Autodesk Inventor part; units mm, degrees
ref_plane "Arbeitsebene1" through (0, 0, 0) normal (0, 1, 0) x (-1, 0, 0)
ref_plane "YZ Plane" through (0, 0, 0) normal (1, 0, 0) x (0, 1, 0)
ref_plane "XY Plane" through (0, 0, 0) normal (0, 0, 1) x (1, 0, 0)
sketch "Skizze1" plane through (0, 0, 0) normal (0, 0, 1) x (1, 0, 0)
  line L0 (-2.6307, 4) -> (27.3693, 4) construction
  arc A0 (0, 0) -> (24.7386, 0) centre (12.3693, 4) ccw
  circle A1 centre (12.3693, 4) radius 5.5
  line L1 (17.8693, 4) -> (24.7386, 0)
  line L2 (6.8693, 4) -> (0, 0)
  line L3 (6.9669, 5.0312) -> (8.4403, 12.75)
  line L4 (17.7718, 5.0312) -> (16.2984, 12.75)
  arc A2 (16.2984, 12.75) -> (8.4403, 12.75) centre (12.3693, 12) ccw
  dimension "d2" = 26
  dimension "d3" = 11
  dimension "d4" = 4
  dimension "d5" = 4
  dimension "d6" = 8
extrude "Extrusion1" add sketch "Skizze1" along normal blind 6.5
sketch "Skizze2" plane through (0, 0, 6.5) normal (0, 0, 1) x (1, 0, 0)
  arc A0 (17.8693, 4) -> (17.7718, 5.0312) centre (12.3693, 4) ccw
  line L0 (17.7718, 5.0312) -> (16.2984, 12.75)
  arc A1 (16.2984, 12.75) -> (8.4403, 12.75) centre (12.3693, 12) ccw
  line L1 (8.4403, 12.75) -> (6.9669, 5.0312)
  arc A2 (6.9669, 5.0312) -> (6.8693, 4) centre (12.3693, 4) ccw
  line L2 (6.8693, 4) -> (0, 0)
  arc A3 (0, 0) -> (24.7386, 0) centre (12.3693, 4) ccw
  line L3 (24.7386, 0) -> (17.8693, 4)
  circle A4 centre (12.3693, 4) radius 4
  dimension "d9" = 8
extrude "Extrusion2" cut sketch "Skizze2" against normal up to surface (6.5 mm away) contours A4
sketch "Skizze3" plane through (0, 0, 6.5) normal (0, 0, 1) x (1, 0, 0)
  circle A0 centre (12.3693, 4) radius 4
  point P0 (0, 0)
  point P1 (12.3693, 12)
  dimension "d12" = 8
hole "Bohrung1" at (12.3693, 12, 6.5) direction (0, 0, -1) diameter 2.459 depth 6.5 counterbore diameter 4 counterbore depth 0.5
ref_plane "Arbeitsebene1" through (0, 0, 0) normal (0, 1, 0) x (-1, 0, 0)
sketch "Skizze4" plane through (0, 0, 0) normal (0, 1, 0) x (-1, 0, 0)
  line L0 (0, 6.5) -> (-24.7386, 6.5)
  line L1 (0, 0) -> (-24.7386, 0)
  line L2 (-24.7386, 0) -> (-24.7386, 6.5)
  line L3 (0, 6.5) -> (-24.7386, 6.5)
  line L4 (0, 0) -> (0, 6.5)
  point P0 (-12.3693, 6.5)
  point P1 (-10.2818, 3.5)
  point P2 (-12.3693, 6.5)
  dimension "d25" = 3
  dimension "d26" = 14.4568
hole "Bohrung2" at (10.2818, 0, 3.5) direction (0, -1, 0) diameter 3 end through all
properties part number "Kurbel" material "Stahl, galvanisiert"
The model under review builds one solid part; all positions refer to its coordinate system, in mm. A direction names the side the tool comes from. Give positions to 0.01 mm unless a question says otherwise; leave off trailing zeros. Order: outer loops, then holes, each group sorted by start corner. A loop starts at its lowest first (then second) coordinate and runs counter-clockwise, first axis right, second up. Notation, with made-up numbers: (74, 33.5) -> (100, 33.5) arc R16 ccw to (100, 42.5) -> close; hole circle Ø9 at (4.5, 61.5). An arc over 180 degrees is marked (long way). Write item = value, one per line. Start each with the question number.
(1) Draft analysis for pull direction X (two halves, no side actions). For faces 4 (the flat face through (21.3, 2, 3.2)), 5 (the flat face through (12, -2, 0)), 6 (the flat face through (10, 0, 3)), state which applies: +X half, -X half, draft (parallel to the pull), parting line (faces both ways), or undercut.
(2) For pin 1 Ø2 at (x, y) = (12.37, 12) entering from +Z; pin 2 Ø0.9 at (x, z) = (10.5, 4) entering from -Y; pin 3 Ø2.5 at (x, z) = (10.28, 3.5) entering from +Y; pin 4 Ø1 at (y, z) = (4, 3.5) entering from +X, all flat-tipped, find the tip position at first contact; note any pin that passes through.
(3) Tool access review of faces 1 (the cylindrical face through (11.613, -4.556, 4.192)), 2 (the cylindrical face through (12.3, 16, 3.2)), 3 (the cylindrical face through (11.018, 13.474, 6.246)): name each direction out of +Z, -Z, +X, -X, +Y, -Y from which nothing blocks a thin tool from reaching the whole face with its end or side.
(4) For L1, parallel to Y at x = 13.25, z = 6.25; L2, parallel to Y at x = 9.25, z = 1.75; L3, parallel to X at y = -4, z = 3.5, list the stretches that pass through material, from the lowest coordinate up. Write a range as from..to.
(5) Take a section at A-A (y = 2). Write out the cut boundary in (x, z), plus the area to 3 significant figures.
(6) Take a section at C-C (y = -2.75). Write out the cut boundary in (x, z).
(7) Take a section at D-D (y = 12). Write out the cut boundary in (x, z), plus the area to 3 significant figures.
(8) Take a section at B-B (z = 3). Write out the cut boundary in (x, y), plus the area to 3 significant figures.
Returned:
q1.face_4 = +X half
q1.face_5 = draft
q1.face_6 = undercut
q2.pin_1 = through
q2.pin_2 = 0
q2.pin_3 = 15.91
q2.pin_4 = 18.73
q3.face_1 = -Y
q3.face_2 = +Z, -Z, +Y
q3.face_3 = +Z
q4.L1 = -8.97..0.1, 7.9..10.2, 13.8..15.9
q4.L2 = -8.62..1.5, 6.5..14.5
q4.L3 = 2.12..8.78, 11.78..22.62
q5.outline = (3.43, 0) -> (8.91, 0) -> (8.91, 6.5) -> (3.43, 6.5) -> close; (15.83, 0) -> (21.3, 0) -> (21.3, 6.5) -> (15.83, 6.5) -> close
q5.area = 71.1 mm²
q6.outline = (1.26, 0) -> (23.48, 0) -> (23.48, 6.5) -> (1.26, 6.5) -> close; hole circle Ø3 at (10.28, 3.5)
q7.outline = (8.3, 0) -> (11.14, 0) -> (11.14, 6) -> (10.37, 6) -> (10.37, 6.5) -> (8.3, 6.5) -> close; (13.6, 0) -> (16.44, 0) -> (16.44, 6.5) -> (14.37, 6.5) -> (14.37, 6) -> (13.6, 6) -> close
q7.area = 36.2 mm²
q8.outline = (0, 0) arc R13 ccw to (8.87, -8.52) -> (8.87, 0) -> (11.7, 0) -> (11.7, -8.98) arc R13 ccw to (24.74, 0) -> (17.87, 4) arc R5.5 ccw to (17.77, 5.03) -> (16.3, 12.75) arc R4 ccw to (8.44, 12.75) -> (6.97, 5.03) arc R5.5 ccw to (6.87, 4) -> close; hole circle Ø8 at (12.37, 4); hole circle Ø2.46 at (12.37, 12)
q8.area = 257 mm²
